Verification items for the finished model (mm, model axes). A direction names the side the tool comes from. Give positions to 0.01 mm unless a question says otherwise; leave off trailing zeros. Order: outer loops, then holes, each group sorted by start corner. A loop starts at its lowest first (then second) coordinate and runs counter-clockwise, first axis right, second up. Notation, with made-up numbers: (-10, 61) - (-2, 61) arc R21 cw to (-2, 71) - close; hole circle Ø6 at (76.25, -7). An arc over 180 degrees is marked (long way). Answer as a JSON object with one key per item and string values. Group by question number.
(1) Thickness scan on line 1 (Z direction, x = 8.5, y = 32) (3 decimals); line 2 (Z direction, x = 64, y = 2.5) (3 decimals); line 3 (Y direction, x = 44.5, z = 54.5). Record the ranges inside material, lowest first.
(2) Access from +Z, -Z, +X, -X, +Y, -Y to the whole of each face (thin tool, end or side, straight path). Record for faces 4 (the face through (46, -25.4, 42)), 5 (the face through (86, 0, 38.1)), 6 (the face through (-3, -7.938, 30)), 7 (the face through (22.225, 17, 18)), 8 (the face through (39.464, -61.59, 0.133)).
(3) Depth check by flat-ended pin: pin 1 Ø18.5 at (y, z) = (-24.5, 8.5) entering from +X (3 decimals); pin 2 Ø8.5 at (y, z) = (19.5, 17.5) entering from -X (3 decimals); pin 3 Ø15.5 at (x, z) = (40, 44.5) entering from -Y; pin 4 Ø10 at (x, y) = (84.5, 32) entering from +Z. Enter the tip coordinate at first touch or a pass-through.
(4) Section check A-A (z = -1). Record the boundary of the cut face in (x, y) (3 decimals).
(5) Section check B-B (x = 64.5). Record the boundary of the cut face in (y, z) (3 decimals), then the cut area to 3 significant figures.
(6) Mould release check, pull along X, two halves, no side actions. Record for faces 1 (the face through (-39.464, 61.59, -0.133)), 2 (the face through (45.8, -0.4, 38.1)), 3 (the face through (-3, 7.938, 30)): +X half, -X half, draft (parallel to the pull), parting line (faces both ways), or undercut.
(7) Section check C-C (y = -49.5). Record the boundary of the cut face in (x, z) (3 decimals).
```python
from build123d import *

# Parameters (mm, degrees)
F1_DEPTH = 63.5
F0_W     = 25.4
F0_H     = 19.05
F2_DEPTH = 25.4
F3_DEPTH = 7.9375
F5_R     = 6.35


with BuildPart() as f1:
    # F0 (on Front) → F1 (new body, symmetric)
    with BuildSketch(Plane.XZ):
        Polygon((-41.275, -9.525), (41.275, -9.525), (41.275, 9.525), (22.225, 9.525), (-41.275, 9.525), align=None)
    extrude(amount=F1_DEPTH, both=True)

    # F0 (on Front) → F2 (join, symmetric)
    with BuildSketch(Plane.XZ):
        with Locations((73.025, 52.4002)):
            Rectangle(F0_W, F0_H)
        with BuildLine():
            Line((22.225, 9.525), (41.275, 9.525))
            Line((41.275, 9.525), (41.275, 27.0002))
            ThreePointArc((41.275, 27.0002), (45.9246798487, 38.2255201513), (57.15, 42.8752))
            Line((57.15, 42.8752), (60.325, 42.8752))
            Line((60.325, 42.8752), (60.325, 61.9252))
            Line((60.325, 61.9252), (57.15, 61.9252))
            add(Edge.make_bspline(
                [(56.0893351364, 61.9090902007), (56.4456274425, 61.9167445082), (56.7992126462, 61.9221202842), (57.15, 61.9252)],
                knots=[110.3910816618, 110.3910816618, 110.3910816618, 110.3910816618, 111.5045361635, 111.5045361635, 111.5045361635, 111.5045361635], degree=3))
            ThreePointArc((56.0893351364, 61.9090902007), (32.082098758, 51.3180114212), (22.225, 27.0002))
            Line((22.225, 27.0002), (22.225, 9.525))
        make_face()
    extrude(amount=F2_DEPTH, both=True)

    # F0 (on Front) → F3 (join, symmetric)
    with BuildSketch(Plane.XZ):
        with BuildLine():
            add(Edge.make_bspline(
                [(-41.275, 9.525), (-41.167300735, 37.9949573937), (20.7654911939, 61.1502201412), (56.0893351364, 61.9090902007)],
                knots=[0, 0, 0, 0, 110.3910816618, 110.3910816618, 110.3910816618, 110.3910816618], degree=3))
            Line((-41.275, 9.525), (22.225, 9.525))
            Line((22.225, 9.525), (22.225, 27.0002))
            ThreePointArc((22.225, 27.0002), (32.082098758, 51.3180114212), (56.0893351364, 61.9090902007))
        make_face()
    extrude(amount=F3_DEPTH, both=True)

    # F0 (on Front) → F4 (revolve)
    with BuildSketch(Plane.XZ):
        Polygon((85.725, 61.9252), (85.725, 42.8752), (85.725, 38.1), (111.125, 38.1), (111.125, 66.675), (85.725, 66.675), align=None)
    revolve(axis=Axis((85.725, 0, 52.3875), (0, 0, 1)))

    # F5
    f5_edges = [f1.edges().sort_by_distance(p)[0] for p in [
        (-41.275, -63.5, 0),
        (41.275, -63.5, 0),
        (41.275, 63.5, 0),
        (-41.275, 63.5, 0),
    ]]
    fillet(f5_edges, radius=F5_R)


solid = f1.part
```
Solutions:
{
 "1": {"line 1": "z = -9.525 to 9.525", "line 2": "z = 38.1 to 66.675", "line 3": "y = -25.4 to 25.4"},
 "2": {"face 4": "+Z, +X, -X, -Y", "face 5": "-Z, +X, +Y, -Y", "face 6": "+Z, -X, -Y", "face 7": "+Z, -X, +Y", "face 8": "+Z, -Z, +X, -Y"},
 "3": {"pin 1": "stops at x = 41.275", "pin 2": "stops at x = 22.225", "pin 3": "stops at y = -25.4", "pin 4": "passes through"},
 "4": {"outline": "(-41.275, -57.15) arc R6.35 ccw to (-34.925, -63.5) - (34.925, -63.5) arc R6.35 ccw to (41.275, -57.15) - (41.275, 57.15) arc R6.35 ccw to (34.925, 63.5) - (-34.925, 63.5) arc R6.35 ccw to (-41.275, 57.15) - close"},
 "5": {"outline": "(-25.4, 42.875) - (-13.952, 42.875) - (-13.952, 38.1) - (13.952, 38.1) - (13.952, 42.875) - (25.4, 42.875) - (25.4, 61.925) - (13.952, 61.925) - (13.952, 66.675) - (-13.952, 66.675) - (-13.952, 61.925) - (-25.4, 61.925) - close", "area": "1,230 mm2"},
 "6": {"face 1": "-X half", "face 2": "undercut", "face 3": "draft"},
 "7": {"outline": "(-41.275, -9.525) - (41.275, -9.525) - (41.275, 9.525) - (-41.275, 9.525) - close"}
}
